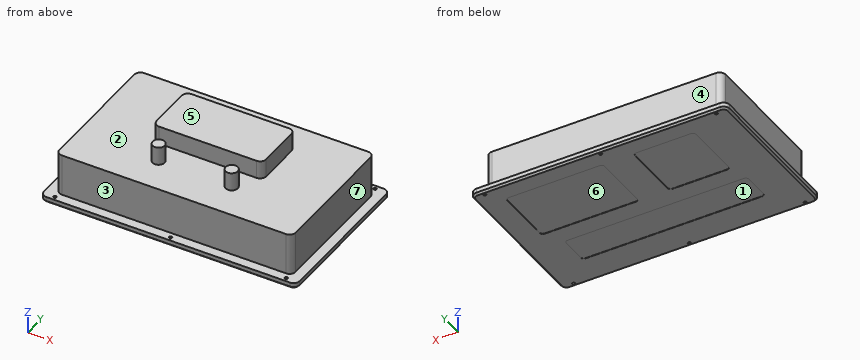
```python
from build123d import *

# Parameters (mm, degrees)
SKETCH_1_W          = 420
SKETCH_1_H          = 260
EXTRUDE_1_DEPTH     = 10
SKETCH_2_W          = 388
SKETCH_2_H          = 228
EXTRUDE_2_DEPTH     = 69
SKETCH_3_R          = 10
SKETCH_3_W          = 180
SKETCH_3_H          = 90
EXTRUDE_3_DEPTH     = 30
SKETCH_4_R          = 2.5
CUT_EXTRUDE_1_DEPTH = 270.964812522
FILLET_1_R          = 10
CUT_EXTRUDE_2_DEPTH = 0.5
CHAMFER_1_SIZE      = 3


with BuildPart() as part:
    # 草图1 → 凸台-拉伸1 (new body)
    with BuildSketch(Plane.XY):
        Rectangle(SKETCH_1_W, SKETCH_1_H)
    extrude(amount=EXTRUDE_1_DEPTH)

    # 草图2 → 凸台-拉伸2 (add)
    with BuildSketch(Plane.XY.offset(10)):
        Rectangle(SKETCH_2_W, SKETCH_2_H)
    extrude(amount=EXTRUDE_2_DEPTH)

    # 草图3 → 凸台-拉伸3 (add)
    with BuildSketch(Plane.XY.offset(79)):
        with Locations(Location((-60, -55, 0), (0, 0, 180))):
            Circle(SKETCH_3_R)
        with Locations(Location((60, -55, 0), (0, 0, 180))):
            Circle(SKETCH_3_R)
        with Locations((0, 25)):
            Rectangle(SKETCH_3_W, SKETCH_3_H)
    extrude(amount=EXTRUDE_3_DEPTH)

    # 草图4 → 切除-拉伸1 (cut, through all)
    with BuildSketch(Plane(origin=(0, 0, 0), x_dir=(-1, 0, 0), z_dir=(0, 0, -1))):
        with Locations((-190, 123.5)):
            Circle(SKETCH_4_R)
        with Locations((0, 123.5)):
            Circle(SKETCH_4_R)
        with Locations((190, 123.5)):
            Circle(SKETCH_4_R)
        with Locations((190, -123.5)):
            Circle(SKETCH_4_R)
        with Locations((0, -123.5)):
            Circle(SKETCH_4_R)
        with Locations((-190, -123.5)):
            Circle(SKETCH_4_R)
    extrude(amount=-CUT_EXTRUDE_1_DEPTH, mode=Mode.SUBTRACT)

    # 圆角1
    fillet_1_edges = [part.edges().sort_by_distance(p)[0] for p in [
        (194, -114, 44.5),
        (194, 114, 44.5),
        (-194, 114, 44.5),
        (-194, -114, 44.5),
        (90, -20, 94),
        (90, 70, 94),
        (-90, 70, 94),
        (-90, -20, 94),
        (210, -130, 5),
        (-210, -130, 5),
        (-210, 130, 5),
        (210, 130, 5),
    ]]
    fillet(fillet_1_edges, radius=FILLET_1_R)

    # 草图5 → 切除-拉伸2 (cut)
    with BuildSketch(Plane(origin=(0, 0, 0), x_dir=(-1, 0, 0), z_dir=(0, 0, -1))):
        with BuildLine():
            Line((-165, 0), (-15, 0))
            ThreePointArc((-15, 0), (-11.464466094, 1.464466094), (-10, 5))
            Line((-10, 5), (-10, 95))
            ThreePointArc((-10, 95), (-11.464466094, 98.535533906), (-15, 100))
            Line((-15, 100), (-165, 100))
            ThreePointArc((-165, 100), (-168.535533906, 98.535533906), (-170, 95))
            Line((-170, 95), (-170, 5))
            ThreePointArc((-170, 5), (-168.535533906, 1.464466094), (-165, 0))
        make_face()
        with BuildLine():
            Line((45, 0), (135, 0))
            ThreePointArc((135, 0), (138.535533906, 1.464466094), (140, 5))
            Line((140, 5), (140, 95))
            ThreePointArc((140, 95), (138.535533906, 98.535533906), (135, 100))
            Line((135, 100), (45, 100))
            ThreePointArc((45, 100), (41.464466094, 98.535533906), (40, 95))
            Line((40, 95), (40, 5))
            ThreePointArc((40, 5), (41.464466094, 1.464466094), (45, 0))
        make_face()
        with BuildLine():
            Line((-145, -80), (145, -80))
            ThreePointArc((145, -80), (148.535533906, -78.535533906), (150, -75))
            Line((150, -75), (150, -35))
            ThreePointArc((150, -35), (148.535533906, -31.464466094), (145, -30))
            Line((145, -30), (-145, -30))
            ThreePointArc((-145, -30), (-148.535533906, -31.464466094), (-150, -35))
            Line((-150, -35), (-150, -75))
            ThreePointArc((-150, -75), (-148.535533906, -78.535533906), (-145, -80))
        make_face()
    extrude(amount=-CUT_EXTRUDE_2_DEPTH, mode=Mode.SUBTRACT)

    # 倒角1
    chamfer_1_edges = [part.edges().sort_by_distance(p)[0] for p in [
        (210, 0, 0),
        (0, -130, 0),
        (-210, 0, 0),
        (0, 130, 0),
        (207.071067812, 127.071067812, 0),
        (-207.071067812, 127.071067812, 0),
        (-207.071067812, -127.071067812, 0),
        (207.071067812, -127.071067812, 0),
    ]]
    chamfer(chamfer_1_edges, length=CHAMFER_1_SIZE)


solid = part.part
```
Geometry: final body of the model. Coordinates: model frame, mm. Face numbers are marked on the shaded views. A direction names the side the tool comes from. Round coordinates to 2 decimals unless told otherwise and drop trailing zeros. Order: outer loops, then holes, each group sorted by start corner. A loop starts at its lowest first (then second) coordinate and runs counter-clockwise, first axis right, second up. Notation, with made-up numbers: (57, 62.5) - (71, 62.5) arc R33 cw to (71, 91.5) - close; hole circle Ø6 at (69, -10.75). An arc over 180 degrees is marked (long way). Write item = value, one per line. Start each with the question number.
Q1. Cut plane D-D on x = 57. Return the cut outline in (y, z), and give its area (3 significant figures).
Q2. Pin query (flat end, axial travel): pin 1 (0.6 mm diameter, centred on y = 65, z = 0.5, fed in from +X); pin 2 (1.5 mm diameter, centred on y = -21, z = 93, fed in from +X); pin 3 (10 mm diameter, centred on y = -8.5, z = 79.5, fed in from +X); pin 4 (20.5 mm diameter, centred on x = -9.5, z = 36, fed in from -Y). Return the tip coordinate at first contact, or that it passes through.
Q3. Cut plane C-C on x = -101. Return the cut outline in (y, z), and give its area (3 significant figures).
Q4. Pull-direction query (X, two-part tool) for the marked faces 5, 6 and 7; classes: +X half, -X half, draft (parallel to the pull), parting line (faces both ways), or undercut.
Q5. Cut plane B-B on z = 73.5. Return the cut outline in (x, y).
Q6. Cut plane A-A on x = -13. Return the cut outline in (y, z), and give its area (3 significant figures).
Q7. Ray query, line 1 (Y direction, x = 0, z = 3); line 2 (Y direction, x = -190, z = 2); line 3 (X direction, y = -79, z = 20.5). Return the intervals inside material, ascending. Write a range as from..to.
Q8. Access query for the marked faces 1, 2, 3 and 4. Directions: +Z, -Z, +X, -X, +Y, -Y. A direction counts if a zero-diameter tool reaches every point of the face in a straight line with its end or side. Return the directions, or none.
Outcome:
q1.outline = (-130, 3) - (-127, 0) - (-80, 0) - (-80, 0.5) - (-30, 0.5) - (-30, 0) - (0, 0) - (0, 0.5) - (100, 0.5) - (100, 0) - (127, 0) - (130, 3) - (130, 10) - (114, 10) - (114, 79) - (70, 79) - (70, 109) - (-20, 109) - (-20, 79) - (-45.46, 79) - (-45.46, 109) - (-64.54, 109) - (-64.54, 79) - (-114, 79) - (-114, 10) - (-130, 10) - close
q1.area = 21,500 mm^2
q2.pin_1 = 207.8
q2.pin_2 = through
q2.pin_3 = 194
q2.pin_4 = -114
q3.outline = (-130, 3) - (-127, 0) - (-80, 0) - (-80, 0.5) - (-30, 0.5) - (-30, 0) - (0, 0) - (0, 0.5) - (100, 0.5) - (100, 0) - (127, 0) - (130, 3) - (130, 10) - (114, 10) - (114, 79) - (-114, 79) - (-114, 10) - (-130, 10) - close
q3.area = 18,200 mm^2
q4.face_5 = draft
q4.face_6 = undercut
q4.face_7 = +X half
q5.outline = (-194, -104) arc R10 ccw to (-184, -114) - (184, -114) arc R10 ccw to (194, -104) - (194, 104) arc R10 ccw to (184, 114) - (-184, 114) arc R10 ccw to (-194, 104) - close
q6.outline = (-130, 3) - (-127, 0) - (-80, 0) - (-80, 0.5) - (-30, 0.5) - (-30, 0) - (127, 0) - (130, 3) - (130, 10) - (114, 10) - (114, 79) - (70, 79) - (70, 109) - (-20, 109) - (-20, 79) - (-114, 79) - (-114, 10) - (-130, 10) - close
q6.area = 21,000 mm^2
q7.line_1 = -130..-126, -121..121, 126..130
q7.line_2 = -129..-126, -121..121, 126..129
q7.line_3 = -194..194
q8.face_1 = -Z
q8.face_2 = +Z
q8.face_3 = +Z, +X, -X, -Y
q8.face_4 = +Z, +X, -X, +Y
